Verification items for the finished model (mm, model axes). Face numbers are marked on the shaded views. A direction names the side the tool comes from. Coordinates: 2 decimals unless noted, no trailing zeros. Order: outer loops, then holes, each group sorted by start corner. A loop starts at its lowest first (then second) coordinate and runs counter-clockwise, first axis right, second up. Notation, with made-up numbers: M 66.5,-26 L 114.5,-26 A9 ccw 114.5,-21 Z; hole C -27.75,6.25 d1. An arc over 180 degrees is marked long. Answer as a JSON object with one key per item and string values. Group by question number.
(1) Cross-section at A-A (z = 25.5). Enter the section's corners in (x, y), plus the area to 3 significant figures.
(2) Material ranges on line 1 (Y direction, x = 0, z = 162.5); line 2 (Z direction, x = 1, y = -6.25); line 3 (X direction, y = 0.25, z = 29), recorded low to high.
(3) Gauge pin test, flat ends, axial feed: pin 1 Ø1.5 at (y, z) = (-2.5, 20) entering from +X; pin 2 Ø3 at (x, z) = (6.5, 52.5) entering from -Y (3 decimals); pin 3 Ø6 at (x, z) = (-5, 80.5) entering from +Y. Record the tip position at first contact, or that the pin passes through.
(4) Access from +Z, -Z, +X, -X, +Y, -Y to the whole of each face (thin tool, end or side, straight path). Record for the marked faces 1, 2 and 3.
from build123d import *

# Parameters (mm, degrees)
F0_R      = 7.5
F1_DEPTH  = 15
F2_R      = 8
F3_DEPTH  = 100
F4_R      = 7.5
F5_DEPTH  = 15
F6_R      = 6
F7_DEPTH  = 25
F8_R      = 5
F9_DEPTH  = 12
F11_D     = 5
F11_DEPTH = 12
F11_TIP   = 1.5021515476


with BuildPart() as f1:
    # F0 (on Top) → F1 (new body)
    with BuildSketch(Plane.XY):
        Circle(F0_R)
    extrude(amount=F1_DEPTH)

    # F2 (on face) → F3 (join)
    with BuildSketch(Plane.XY.offset(15)):
        Circle(F2_R)
    extrude(amount=F3_DEPTH)

    # F4 (on face) → F5 (join)
    with BuildSketch(Plane.XY.offset(115)):
        Circle(F4_R)
    extrude(amount=F5_DEPTH)

    # F6 (on face) → F7 (join)
    with BuildSketch(Plane.XY.offset(130)):
        Circle(F6_R)
    extrude(amount=F7_DEPTH)

    # F8 (on face) → F9 (join)
    with BuildSketch(Plane.XY.offset(155)):
        Circle(F8_R)
    extrude(amount=F9_DEPTH)

    # F11
    with Locations(Plane.XY.offset(167)):
        with Locations((0, 0)):
            Hole(F11_D / 2, depth=F11_DEPTH)
            with Locations((0, 0, -(F11_DEPTH + F11_TIP / 2))):  # 118° drill point
                Cone(0, F11_D / 2, F11_TIP, mode=Mode.SUBTRACT)


solid = f1.part
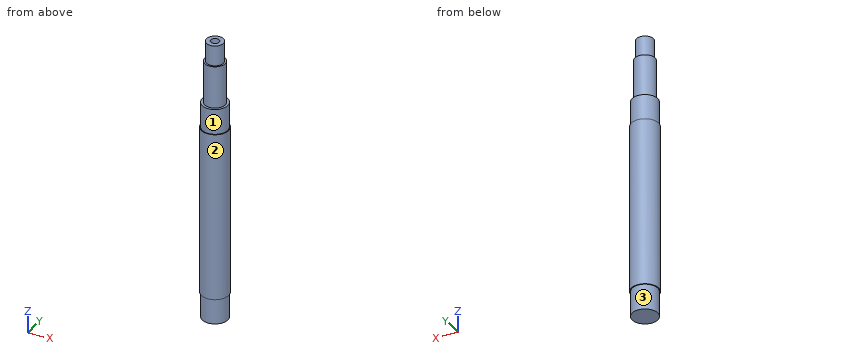
Taken from the geometry:
{
 "1": {"outline": "C 0,0 d16", "area": "201 mm²"},
 "2": {"line 1": "y = -5 to -2.5, 2.5 to 5", "line 2": "z = 0 to 130", "line 3": "x = -8 to 8"},
 "3": {"pin 1": "stops at x = 7.81", "pin 2": "stops at y = -6.245", "pin 3": "stops at y = 7.75"},
 "4": {"face 1": "+Z", "face 2": "+Z, -Z", "face 3": "-Z"}
}
